Build history of the part. All positions in model axes, mm. A direction names the side the tool comes from. Round coordinates to 2 decimals unless told otherwise and drop trailing zeros. Loops run counter-clockwise (first coordinate to the right, second up) from the corner with the lowest first, then second, coordinate; pieces in that order, holes last. Notation, with made-up numbers: (73, 12.5) - (119, 12.5) arc R25 cw to (119, 50.5) - close; hole circle Ø4 at (14, 40). An arc over 180 degrees is marked (long way). Use one line per item in the form item = value. Start each with the question number.
Q1. Saw through at C-C (y = -62.1). Give the cut face in (x, z), then the cut area to 3 significant figures.
Q2. Saw through at D-D (z = 23). Give the cut face in (x, y), then the cut area to 3 significant figures.
Q3. Saw through at B-B (x = -6). Give the cut face in (y, z), then the cut area to 3 significant figures.
Q4. Saw through at A-A (z = 128.3). Give the cut face in (x, y).
Q5. Mould opens along Y. For faces 1 (the face through (-6, 0, 68)), 2 (the face through (-1, -28, 0)), 3 (the face through (-6, -60, 92)), 4 (the face through (-0.76, -47.097, 29.538)) say: released by +Y, released by -Y, zero draft, split by the parting line, or undercut.
Q6. 3-axis set-ups, long thin cutter, end or side, ignore diameter. For faces 5 (the face through (-5, -59, 50)), 6 (the face through (0, -41, 66)), 7 (the face through (-0.8, -90.5, 22.9)), 8 (the face through (-6, -1.5, 68)), 9 (the face through (-5.71, -59.26, 126.07)): which of +Z, -Z, +X, -X, +Y, -Y reach the whole face in a straight line?
Q7. Pin check, flat tips, straight feed: pin 1 (4 mm diameter, centred on x = -6, z = 128.3, fed in from -Y); pin 2 (1.2 mm diameter, centred on x = -1, y = -85.5, fed in from +Z); pin 3 (5 mm diameter, centred on y = -45.1, z = 17.5, fed in from -X). Stop position of each tip, or through.
Q8. Drill centre lines: line 1 (Y direction, x = -6, z = 84); line 2 (Y direction, x = -1, z = 44.2); line 3 (Y direction, x = -1.15, z = 56.2). Where is each one in solid material? Low to high.
```python
from build123d import *

# Parameters (mm, degrees)
SKETCH_1_W                        = 1.5
SKETCH_1_H                        = 100
SM_BASE_FLANGE_1_DEPTH            = 134.6
SKETCH_6_R                        = 2.25
SKETCH_6_R_2                      = 2.5
SKETCH_6_R_3                      = 6
SKETCH_6_W                        = 89.6
SKETCH_6_H                        = 40
SKETCH_6_W_2                      = 10
SKETCH_6_H_2                      = 14
CUT_EXTRUDE_1_DEPTH               = 10
SKETCH_10_W                       = 5
SKETCH_10_H                       = 2.2
CUT_EXTRUDE_2_DEPTH               = 10
SM_EDGE_FLANGE_2_STRIP_W          = 7.4732
SM_EDGE_FLANGE_2_STRIP_H          = 1.5
SM_EDGE_FLANGE_2_STRIP_CUT_DEPTH  = 84.6
SM_EDGE_FLANGE_2_RELIEF_W         = 8.2232
SM_EDGE_FLANGE_2_RELIEF_H         = 0.75
SM_EDGE_FLANGE_2_RELIEF_CUT_DEPTH = 1.5
SM_EDGE_FLANGE_2_DEPTH            = 84.6
SM_EDGE_FLANGE_3_STRIP_W          = 7.4732
SM_EDGE_FLANGE_3_STRIP_H          = 1.5
SM_EDGE_FLANGE_3_STRIP_CUT_DEPTH  = 134.6
SM_EDGE_FLANGE_3_DEPTH            = 134.6
CUT_EXTRUDE_3_DEPTH               = 10
SKETCH_18_R                       = 2.25
CUT_EXTRUDE_4_DEPTH               = 10


# Sheet-metal steps are written as plain solids
with BuildPart() as part:
    # Sketch 1 → 基体-法兰1 (new body)
    with BuildSketch(Plane.XY):
        with Locations((-0.75, -50)):
            Rectangle(SKETCH_1_W, SKETCH_1_H)
    extrude(amount=SM_BASE_FLANGE_1_DEPTH)

    # 草图6 → 切除-拉伸1 (cut)
    with BuildSketch(Plane.ZY.offset(1.5)):
        with Locations((17.5, -45.10094434)):
            Circle(SKETCH_6_R)
        with Locations((28.5, -45.10094434)):
            Circle(SKETCH_6_R)
        with Locations((44.2, -33.4)):
            Circle(SKETCH_6_R)
        with Locations((56.2, -33.4)):
            Circle(SKETCH_6_R)
        with Locations((44.2, -40.9)):
            Circle(SKETCH_6_R_2)
        with Locations((56.2, -40.9)):
            Circle(SKETCH_6_R_2)
        with Locations((64.7, -33.4)):
            Circle(SKETCH_6_R_2)
        with Locations((89.6, -47.1)):
            Circle(SKETCH_6_R_3)
        with Locations((23, -62.1)):
            Circle(SKETCH_6_R_3)
        with Locations((89.8, -80)):
            Rectangle(SKETCH_6_W, SKETCH_6_H)
        with Locations((5, -72)):
            Rectangle(SKETCH_6_W_2, SKETCH_6_H_2)
        with BuildLine():
            Line((20, -82.5), (20, -87.5))
            ThreePointArc((20, -87.5), (23, -90.5), (26, -87.5))
            Line((26, -87.5), (26, -82.5))
            ThreePointArc((26, -82.5), (23, -79.5), (20, -82.5))
        make_face()
    extrude(amount=-CUT_EXTRUDE_1_DEPTH, mode=Mode.SUBTRACT)

    # 草图10 → 切除-拉伸2 (cut)
    with BuildSketch(Plane.ZY.offset(1.5)):
        with Locations((47.5, -58.9)):
            Rectangle(SKETCH_10_W, SKETCH_10_H)
    extrude(amount=-CUT_EXTRUDE_2_DEPTH, mode=Mode.SUBTRACT)

    # 边线-法兰2 strip (across the edge) → 边线-法兰2 strip cut (cut)
    with BuildSketch(Plane(origin=(-1.5, -60, 50), x_dir=(0, 1, 0), z_dir=(0, 0, 1))):
        with Locations((-1.5, -0.75)):
            Rectangle(SM_EDGE_FLANGE_2_STRIP_W, SM_EDGE_FLANGE_2_STRIP_H)
    extrude(amount=SM_EDGE_FLANGE_2_STRIP_CUT_DEPTH, mode=Mode.SUBTRACT)

    # 边线-法兰2 relief (on the sheet) → 边线-法兰2 relief cut (cut)
    with BuildSketch(Plane(origin=(-1.5, -57.7634, 50), x_dir=(0, 1, 0), z_dir=(-1, 0, 0))):
        with Locations((-3.3616, 0.375)):
            Rectangle(SM_EDGE_FLANGE_2_RELIEF_W, SM_EDGE_FLANGE_2_RELIEF_H)
    extrude(amount=-SM_EDGE_FLANGE_2_RELIEF_CUT_DEPTH, mode=Mode.SUBTRACT)

    # 边线-法兰2 section (across the edge) → 边线-法兰2 (add)
    with BuildSketch(Plane(origin=(-1.5, -60, 50), x_dir=(0, 1, 0), z_dir=(0, 0, 1))):
        with BuildLine():
            Line((0, 0.7366), (0, 8.5))
            Line((0, 8.5), (1.5, 8.5))
            Line((1.5, 8.5), (1.5, 0.7366))
            ThreePointArc((1.5, 0.7366), (1.715745145, 0.215745145), (2.2366, 0))
            Line((2.2366, 0), (2.2366, -1.5))
            ThreePointArc((2.2366, -1.5), (0.655084973, -0.844915027), (0, 0.7366))
        make_face()
    extrude(amount=SM_EDGE_FLANGE_2_DEPTH)

    # 边线-法兰3 strip (across the edge) → 边线-法兰3 strip cut (cut)
    with BuildSketch(Plane(origin=(-1.5, 0, 134.6), x_dir=(0, -1, 0), z_dir=(0, 0, -1))):
        with Locations((-1.5, -0.75)):
            Rectangle(SM_EDGE_FLANGE_3_STRIP_W, SM_EDGE_FLANGE_3_STRIP_H)
    extrude(amount=SM_EDGE_FLANGE_3_STRIP_CUT_DEPTH, mode=Mode.SUBTRACT)

    # 边线-法兰3 section (across the edge) → 边线-法兰3 (add)
    with BuildSketch(Plane(origin=(-1.5, 0, 134.6), x_dir=(0, -1, 0), z_dir=(0, 0, -1))):
        with BuildLine():
            Line((0, 0.7366), (0, 8.5))
            Line((0, 8.5), (1.5, 8.5))
            Line((1.5, 8.5), (1.5, 0.7366))
            ThreePointArc((1.5, 0.7366), (1.715745145, 0.215745145), (2.2366, 0))
            Line((2.2366, 0), (2.2366, -1.5))
            ThreePointArc((2.2366, -1.5), (0.655084973, -0.844915027), (0, 0.7366))
        make_face()
    extrude(amount=SM_EDGE_FLANGE_3_DEPTH)

    # 草图17 → 切除-拉伸3 (cut)
    with BuildSketch(Plane.XZ.offset(1.5)):
        with BuildLine():
            Line((-8.25, 17.3), (-8.25, 32.3))
            ThreePointArc((-8.25, 32.3), (-6, 34.55), (-3.75, 32.3))
            Line((-3.75, 32.3), (-3.75, 17.3))
            ThreePointArc((-3.75, 17.3), (-6, 15.05), (-8.25, 17.3))
        make_face()
        with BuildLine():
            Line((-3.75, 117.3), (-3.75, 102.3))
            ThreePointArc((-3.75, 102.3), (-6, 100.05), (-8.25, 102.3))
            Line((-8.25, 102.3), (-8.25, 117.3))
            ThreePointArc((-8.25, 117.3), (-6, 119.55), (-3.75, 117.3))
        make_face()
    extrude(amount=-CUT_EXTRUDE_3_DEPTH, mode=Mode.SUBTRACT)

    # 草图18 → 切除-拉伸4 (cut)
    with BuildSketch(Plane.XZ.offset(60)):
        with Locations((-6, 56.3)):
            Circle(SKETCH_18_R)
        with Locations(Location((-6, 128.3, 0), (0, 0, 180))):
            Circle(SKETCH_18_R)
    extrude(amount=-CUT_EXTRUDE_4_DEPTH, mode=Mode.SUBTRACT)


solid = part.part
```
Report:
q1.outline = (-1.5, 0) - (0, 0) - (0, 17) - (-1.5, 17) - close; (-1.5, 29) - (0, 29) - (0, 45) - (-1.5, 45) - close
q1.area = 49.5 mm²
q2.outline = (-10, -1.5) - (-8.25, -1.5) - (-8.25, 0) - (-10, 0) - close; (-3.75, -1.5) - (-2.24, -1.5) arc R0.74 cw to (-1.5, -2.24) - (-1.5, -56.1) - (0, -56.1) - (0, -2.24) arc R2.24 ccw to (-2.24, 0) - (-3.75, 0) - close; (-1.5, -100) - (0, -100) - (0, -90.5) - (-1.5, -90.5) - close; (-1.5, -79.5) - (0, -79.5) - (0, -68.1) - (-1.5, -68.1) - close
q2.area = 121 mm²
q3.outline = (-60, 50) - (-58.5, 50) - (-58.5, 54.05) - (-60, 54.05) - close; (-60, 58.55) - (-58.5, 58.55) - (-58.5, 126.05) - (-60, 126.05) - close; (-60, 130.55) - (-58.5, 130.55) - (-58.5, 134.6) - (-60, 134.6) - close; (-1.5, 0) - (0, 0) - (0, 15.05) - (-1.5, 15.05) - close; (-1.5, 34.55) - (0, 34.55) - (0, 100.05) - (-1.5, 100.05) - close; (-1.5, 119.55) - (0, 119.55) - (0, 134.6) - (-1.5, 134.6) - close
q3.area = 257 mm²
q4.outline = (-10, -60) - (-8.25, -60) - (-8.25, -58.5) - (-10, -58.5) - close; (-10, -1.5) - (-2.24, -1.5) arc R0.74 cw to (-1.5, -2.24) - (-1.5, -57.76) arc R0.74 cw to (-2.24, -58.5) - (-3.75, -58.5) - (-3.75, -60) - (-2.24, -60) arc R2.24 ccw to (0, -57.76) - (0, -2.24) arc R2.24 ccw to (-2.24, 0) - (-10, 0) - close
q5.face_1 = released by +Y
q5.face_2 = zero draft
q5.face_3 = released by -Y
q5.face_4 = undercut
q6.face_5 = +X, -X, -Y
q6.face_6 = +Z, -Z, +X, +Y, -Y
q6.face_7 = +X, -X
q6.face_8 = +Z, -Z, -X
q6.face_9 = -Y
q7.pin_1 = -1.5
q7.pin_2 = 45
q7.pin_3 = -1.5
q8.line_1 = -60 to -58.5, -1.5 to 0
q8.line_2 = -100 to -43.4, -38.4 to -35.65, -31.15 to -0.37
q8.line_3 = -59.72 to -43.4, -38.4 to -35.65, -31.15 to -0.28
